from build123d import *

# Parameters (mm, degrees)
SKETCH1_W           = 144
SKETCH1_H           = 64
SKETCH1_W_2         = 370
SKETCH1_H_2         = 180
BOSS_EXTRUDE1_DEPTH = 1


with BuildPart() as part:
    # Sketch1 → Boss-Extrude1 (new, symmetric)
    with BuildSketch(Plane.XY):
        with BuildLine():
            Line((-325, 310), (325, 310))
            ThreePointArc((325, 310), (360.355339059, 295.355339059), (375, 260))
            Line((375, 260), (375, -310))
            Line((375, -310), (-375, -310))
            Line((-375, -310), (-375, 260))
            ThreePointArc((-375, 260), (-360.355339059, 295.355339059), (-325, 310))
        make_face()
        with Locations((0, -190)):
            Rectangle(SKETCH1_W, SKETCH1_H, mode=Mode.SUBTRACT)
        with Locations((0, -43)):
            Rectangle(SKETCH1_W_2, SKETCH1_H_2, mode=Mode.SUBTRACT)
    extrude(amount=BOSS_EXTRUDE1_DEPTH, both=True)


solid = part.part
Design review of the part built by this model. Coordinates are the model's own, in mm. Coordinates: 2 decimals unless noted, no trailing zeros. Loops run counter-clockwise (first coordinate to the right, second up) from the corner with the lowest first, then second, coordinate; pieces in that order, holes last. Notation, with made-up numbers: (14.5, 54.5) -> (25.5, 54.5) arc R34 ccw to (25.5, 92.5) -> close; hole circle Ø9 at (40.25, 23.25). An arc over 180 degrees is marked (long way). Use a Markdown table: item, result. Add a question column.
Item 1: Wall thickness on L1, parallel to Y at x = 50, z = -0.3; L2, parallel to Y at x = -117, z = 0.9; L3, parallel to X at y = 37.5, z = 0.3: over which ranges is each line inside the solid? List them lowest first. Write a range as from..to.
Item 2: We need section B-B, the plane x = -86. Write out the cut boundary in (y, z).
Item 3: We need section A-A, the plane y = -28. Write out the cut boundary in (x, z).
Item 4: We need section C-C, the plane z = -0.15. Write out the cut boundary in (x, y).
Numbers:
| question | item | result |
|---|---|---|
| 1 | L1 | y = -310..-222, -158..-133, 47..310 |
| 1 | L2 | y = -310..-133, 47..310 |
| 1 | L3 | x = -375..-185, 185..375 |
| 2 | outline | (-310, -1) -> (-133, -1) -> (-133, 1) -> (-310, 1) -> close; (47, -1) -> (310, -1) -> (310, 1) -> (47, 1) -> close |
| 3 | outline | (-375, -1) -> (-185, -1) -> (-185, 1) -> (-375, 1) -> close; (185, -1) -> (375, -1) -> (375, 1) -> (185, 1) -> close |
| 4 | outline | (-375, -310) -> (375, -310) -> (375, 260) arc R50 ccw to (325, 310) -> (-325, 310) arc R50 ccw to (-375, 260) -> close; hole (-185, -133) -> (185, -133) -> (185, 47) -> (-185, 47) -> close; hole (-72, -222) -> (72, -222) -> (72, -158) -> (-72, -158) -> close |
